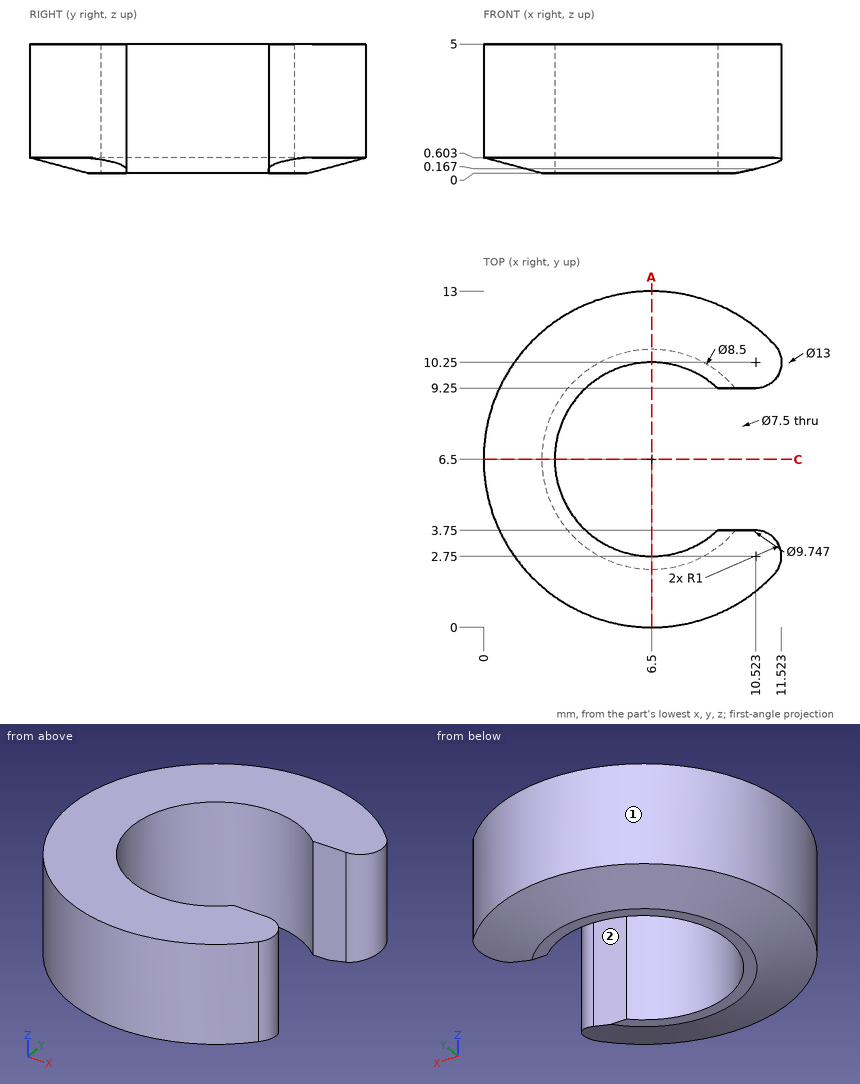
Input: dimensioned drawing with shaded views. Units: mm. Origin: part minimum x, y, z. A direction names the side the tool comes from. Give positions to 0.01 mm unless a question says otherwise; leave off trailing zeros. Loops run counter-clockwise (first coordinate to the right, second up) from the corner with the lowest first, then second, coordinate; pieces in that order, holes last. Notation, with made-up numbers: (24.5, 71) -> (54.5, 71) arc R18 ccw to (54.5, 92) -> close; hole circle Ø11 at (53.25, -15). An arc over 180 degrees is marked (long way). Use a Markdown table: item, result. Add a question column.
1) First-contact query: pin 1 (6 mm diameter, centred on x = 6.5, y = 6.5, fed in from +Z); pin 2 (3 mm diameter, centred on y = 10, z = 3, fed in from -X) (1 decimal); pin 3 (1.6 mm diameter, centred on x = 10, z = 2.5, fed in from +Y); pin 4 (3 mm diameter, centred on x = 8.5, z = 2.5, fed in from +Y). Flat tips, straight axial feed; report the tip coordinate or a pass-through.
2) Section query C-C, the plane y = 6.5. Return the cut outline in (x, z), then the cut area to 3 significant figures.
3) Line query: line 1 along Y through (x, z) = (6.5, 3.4); line 2 along Y through (x, z) = (4.5, 3.8) (1 decimal); line 3 along X through (y, z) = (11.25, 4.85) (1 decimal). Output: solid intervals per line, ascending. Write a range as [from, to].
4) Reachability of the marked faces 1 and 2 from +Z, -Z, +X, -X, +Y, -Y: full face, straight path, thin tool, end or side. Return the list, or none.
5) Section query A-A, the plane x = 6.5. Return the cut outline in (y, z).
Numbers:
| question | item | result |
|---|---|---|
| 1 | pin 1 | passes through |
| 1 | pin 2 | stops at x = 0.3 |
| 1 | pin 3 | stops at y = 12.41 |
| 1 | pin 4 | stops at y = 12.98 |
| 2 | outline | (0, 0.6) -> (2.25, 0) -> (2.75, 0) -> (2.75, 5) -> (0, 5) -> close |
| 2 | area | 13.1 mm2 |
| 3 | line 1 | y = [0, 2.75], [10.25, 13] |
| 3 | line 2 | y = [0.3, 3.3], [9.7, 12.7] |
| 3 | line 3 | x = [2.1, 10.9] |
| 4 | face 1 | +Z, -Z |
| 4 | face 2 | +Z, -Z, +X |
| 5 | outline | (0, 0.6) -> (2.25, 0) -> (2.75, 0) -> (2.75, 5) -> (0, 5) -> close; (10.25, 0) -> (10.75, 0) -> (13, 0.6) -> (13, 5) -> (10.25, 5) -> close |
